Could you check a few things on this model? Use its own coordinates, in mm. Face numbers are marked on the shaded views. Round coordinates to 2 decimals unless told otherwise and drop trailing zeros. Order: outer loops, then holes, each group sorted by start corner. A loop starts at its lowest first (then second) coordinate and runs counter-clockwise, first axis right, second up. Notation, with made-up numbers: (-16, 43) -> (40, 43) arc R22 cw to (40, 56) -> close; hole circle Ø1 at (43, 35.5). An arc over 180 degrees is marked (long way). One line per question, with ' | ' between items.
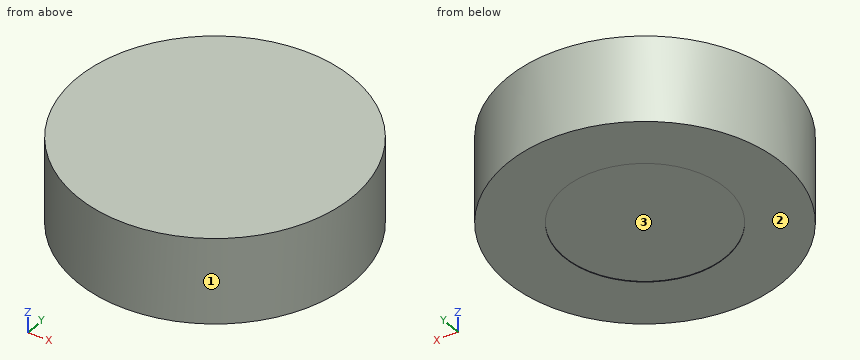
```python
from build123d import *

# Parameters (mm, degrees)
F0_R     = 56.1739618702
F0_R_2   = 32.8963638887
F1_DEPTH = 35.052
F2_DEPTH = 34.798
F0_R_3   = 4.9490742643
F3_DEPTH = 34.798


with BuildPart() as f1:
    # F0 (on Top) → F1 (new body)
    with BuildSketch(Plane.XY):
        Circle(F0_R)
        Circle(F0_R_2, mode=Mode.SUBTRACT)
    extrude(amount=-F1_DEPTH)

    # F0 (on Top) → F2 (join)
    with BuildSketch(Plane.XY):
        Circle(F0_R_2)
        Polygon((24.0832565908, 15.5113956786), (25.4748910012, -13.1010141742), (1.3916344104, -28.6124098528), (-24.0832565908, -15.5113956786), (-25.4748910012, 13.1010141742), (-1.3916344104, 28.6124098528), align=None, mode=Mode.SUBTRACT)
    extrude(amount=-F2_DEPTH)

    # F0 (on Top) → F3 (join)
    with BuildSketch(Plane.XY):
        Polygon((1.3916344104, -28.6124098528), (25.4748910012, -13.1010141742), (24.0832565908, 15.5113956786), (-1.3916344104, 28.6124098528), (-25.4748910012, 13.1010141742), (-24.0832565908, -15.5113956786), align=None)
        Polygon((24.0832565908, 0), (12.0416282954, -20.8567120135), (-12.0416282954, -20.8567120135), (-24.0832565908, 0), (-12.0416282954, 20.8567120135), (12.0416282954, 20.8567120135), align=None, mode=Mode.SUBTRACT)
        Polygon((-12.0416282954, -20.8567120135), (12.0416282954, -20.8567120135), (24.0832565908, 0), (12.0416282954, 20.8567120135), (-12.0416282954, 20.8567120135), (-24.0832565908, 0), align=None)
        Polygon((16.4439717338, 11.0949333309), (17.8304799848, -8.6934305952), (1.3865082509, -19.7883639261), (-16.4439717338, -11.0949333309), (-17.8304799848, 8.6934305952), (-1.3865082509, 19.7883639261), align=None, mode=Mode.SUBTRACT)
        Polygon((1.3865082509, -19.7883639261), (17.8304799848, -8.6934305952), (16.4439717338, 11.0949333309), (-1.3865082509, 19.7883639261), (-17.8304799848, 8.6934305952), (-16.4439717338, -11.0949333309), align=None)
        Polygon((15.2503329708, 0), (7.6251664854, -13.2071757689), (-7.6251664854, -13.2071757689), (-15.2503329708, 0), (-7.6251664854, 13.2071757689), (7.6251664854, 13.2071757689), align=None, mode=Mode.SUBTRACT)
        Polygon((-7.6251664854, -13.2071757689), (7.6251664854, -13.2071757689), (15.2503329708, 0), (7.6251664854, 13.2071757689), (-7.6251664854, 13.2071757689), (-15.2503329708, 0), align=None)
        Polygon((9.7878324796, 4.5358240732), (8.8220551142, -6.2085995387), (-0.9657773653, -10.7444236119), (-9.7878324796, -4.5358240732), (-8.8220551142, 6.2085995387), (0.9657773653, 10.7444236119), align=None, mode=Mode.SUBTRACT)
        Polygon((-0.9657773653, -10.7444236119), (8.8220551142, -6.2085995387), (9.7878324796, 4.5358240732), (0.9657773653, 10.7444236119), (-8.8220551142, 6.2085995387), (-9.7878324796, -4.5358240732), align=None)
        Circle(F0_R_3, mode=Mode.SUBTRACT)
        Circle(F0_R_3)
    extrude(amount=-F3_DEPTH)


solid = f1.part
```
1. If we mould it in two halves opening along X, with no side actions, what happens to the marked faces 1, 2 and 3? For each: pulls with the +X half, pulls with the -X half, needs draft (parallel to the pull), parting line crosses it, or undercut.
From the geometry:
face 1: parting line crosses it | face 2: needs draft | face 3: undercut
2. I want a section at A-A on y = -13. List the corners of the cut face in (x, z) for me.
From the geometry:
outline: (-54.65, -35.05) -> (-30.22, -35.05) -> (-30.22, -34.8) -> (30.22, -34.8) -> (30.22, -35.05) -> (54.65, -35.05) -> (54.65, 0) -> (-54.65, 0) -> close
3. I'm going to push flat-ended pins straight in: pin 1 (19.5 mm diameter, centred on x = -5.5, y = 12.5, fed in from -Z); pin 2 (5 mm diameter, centred on x = 22, z = -17, fed in from -Y); pin 3 (2 mm diameter, centred on x = 18.5, z = -21, fed in from -Y). Where does each tip first touch, or does it pass through?
From the geometry:
pin 1: stops at z = -34.8 | pin 2: stops at y = -52.68 | pin 3: stops at y = -53.38
4. I want a section at D-D on x = -34.5. List the corners of the cut face in (y, z) for me, and give its area (3 significant figures).
From the geometry:
outline: (-44.33, -35.05) -> (44.33, -35.05) -> (44.33, 0) -> (-44.33, 0) -> close | area: 3,110 mm²
5. I want a section at B-B on x = 20.5. List the corners of the cut face in (y, z) for me, and give its area (3 significant figures).
From the geometry:
outline: (-52.3, -35.05) -> (-25.73, -35.05) -> (-25.73, -34.8) -> (25.73, -34.8) -> (25.73, -35.05) -> (52.3, -35.05) -> (52.3, 0) -> (-52.3, 0) -> close | area: 3,650 mm²
6. I want a section at C-C on z = -18.5. List the corners of the cut face in (x, y) for me, and give its area (3 significant figures).
From the geometry:
outline: circle Ø112.35 at (0, 0) | area: 9,910 mm²
7. I need wall thicknesses on probe 1 along Y at (x, z) = (0, -34.85); probe 2 along Z at (x, y) = (2.5, -21.5); probe 3 along Y at (x, z) = (0, -34). Which ranges of each line are inside material? Lowest first, please.
From the geometry:
probe 1: y = -56.17 to -32.9, 32.9 to 56.17 | probe 2: z = -34.8 to 0 | probe 3: y = -56.17 to 56.17
